```python
from build123d import *

# Parameters (mm, degrees)
SKETCH_R         = 2.5
PAD_DEPTH        = 80
SKETCH001_W      = 15
SKETCH001_H      = 10
POCKET_DEPTH     = 16
HOLE_D           = 4.5
HOLE_CSINK_D     = 10
HOLE_CSINK_ANGLE = 90
FILLET_R         = 4
FILLET001_R      = 2
CHAMFER_SIZE2    = 6
CHAMFER_SIZE     = 3
CHAMFER001_SIZE2 = 6
CHAMFER001_SIZE  = 3
FILLET002_R      = 1
FILLET003_R      = 1
FILLET004_R      = 2


with BuildPart() as part:
    # Sketch → Pad (new body)
    with BuildSketch(Plane.XY):
        Polygon((0, 0), (0, 15), (8.325291, 15), (16, 8), (30, 8), (30, 0), align=None)
        with Locations((6, 9)):
            Circle(SKETCH_R, mode=Mode.SUBTRACT)
    extrude(amount=PAD_DEPTH)

    # Sketch001 (on Face1 of Pad) → Pocket (cut)
    with BuildSketch(Plane(origin=(0, 0, 0), x_dir=(0, -1, 0), z_dir=(-1, 0, 0))):
        with Locations((-7.5, 15)):
            Rectangle(SKETCH001_W, SKETCH001_H)
        with Locations((-7.5, 35)):
            Rectangle(SKETCH001_W, SKETCH001_H)
        with Locations((-7.5, 55)):
            Rectangle(SKETCH001_W, SKETCH001_H)
        with Locations((-7.5, 75)):
            Rectangle(SKETCH001_W, SKETCH001_H)
    extrude(amount=-POCKET_DEPTH, mode=Mode.SUBTRACT)

    # Hole (through all)
    with Locations(Plane(origin=(0, 8, 0), x_dir=(-1, 0, 0), z_dir=(0, 1, 0))):
        with Locations((-22.5, 70), (-22.5, 50), (-22.5, 30), (-22.5, 10)):
            CounterSinkHole(HOLE_D / 2, HOLE_CSINK_D / 2, counter_sink_angle=HOLE_CSINK_ANGLE)

    # Fillet
    fillet_edges = [part.edges().sort_by_distance(p)[0] for p in [
        (0, 15, 5),
        (0, 15, 25),
        (0, 15, 45),
        (0, 15, 65),
    ]]
    fillet(fillet_edges, radius=FILLET_R)

    # Fillet001
    fillet001_edges = [part.edges().sort_by_distance(p)[0] for p in [
        (8.325291, 15, 5),
        (8.325291, 15, 25),
        (8.325291, 15, 45),
        (8.325291, 15, 65),
    ]]
    fillet(fillet001_edges, radius=FILLET001_R)

    # Chamfer
    chamfer_edges = [part.edges().sort_by_distance(p)[0] for p in [
        (0, 0, 25),
        (0, 0, 45),
        (0, 0, 65),
    ]]
    chamfer_side = part.faces().sort_by_distance((17.359651, 0, 38.113633))[0]
    chamfer(chamfer_edges, length=CHAMFER_SIZE, length2=CHAMFER_SIZE2, reference=chamfer_side)

    # Chamfer001
    chamfer001_edges = [part.edges().sort_by_distance(p)[0] for p in [
        (0, 0, 5),
    ]]
    chamfer001_side = part.faces().sort_by_distance((18.248211, 0, 37.727814))[0]
    chamfer(chamfer001_edges, length=CHAMFER001_SIZE, length2=CHAMFER001_SIZE2, reference=chamfer001_side)

    # Fillet002
    fillet002_edges = [part.edges().sort_by_distance(p)[0] for p in [
        (16, 8, 5),
        (16, 8, 25),
        (16, 8, 45),
        (16, 8, 65),
    ]]
    fillet(fillet002_edges, radius=FILLET002_R)

    # Fillet003
    fillet003_edges = [part.edges().sort_by_distance(p)[0] for p in [
        (16, 4, 10),
        (16, 4, 30),
        (16, 4, 50),
        (16, 4, 70),
        (16, 4, 80),
        (16, 4, 20),
        (16, 4, 40),
        (16, 4, 60),
    ]]
    fillet(fillet003_edges, radius=FILLET003_R)

    # Fillet004
    fillet004_edges = [part.edges().sort_by_distance(p)[0] for p in [
        (30, 4, 0),
        (30, 4, 80),
    ]]
    fillet(fillet004_edges, radius=FILLET004_R)


solid = part.part
```
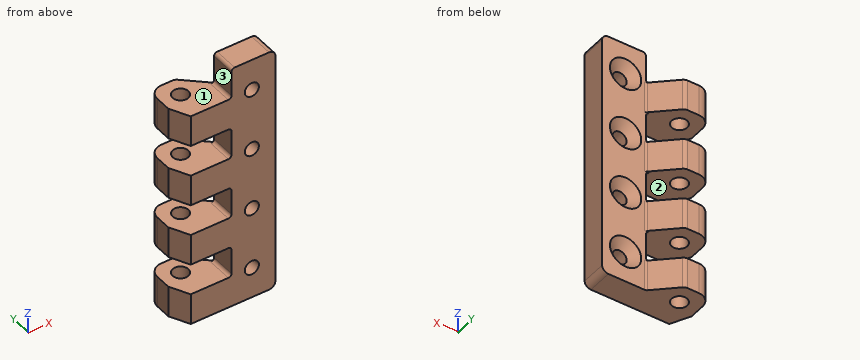
For this review, take the finished solid that the model builds, in its own axes (mm). Face numbers are marked on the shaded views. Round coordinates to 2 decimals unless told otherwise and drop trailing zeros. Write each loop counter-clockwise with the first axis right and the second up, starting at its lowest first coordinate (ties: lowest second). Pieces come first, ordered by that corner, then holes. Notation, with made-up numbers: (-31, 48) - (20, 48) arc R16 ccw to (20, 55) - close; hole circle Ø11 at (-34, 41.5). An arc over 180 degrees is marked (long way). Answer as a JSON object with one key per item and string values.
1. We need section A-A on x = 22.5. Give the boundary of the cut face in (y, z).
Response values:
{"outline": "(0, 0) - (8, 0) - (8, 5) - (5.25, 7.75) - (0, 7.75) - close; (0, 12.25) - (5.25, 12.25) - (8, 15) - (8, 25) - (5.25, 27.75) - (0, 27.75) - close; (0, 32.25) - (5.25, 32.25) - (8, 35) - (8, 45) - (5.25, 47.75) - (0, 47.75) - close; (0, 52.25) - (5.25, 52.25) - (8, 55) - (8, 65) - (5.25, 67.75) - (0, 67.75) - close; (0, 72.25) - (5.25, 72.25) - (8, 75) - (8, 80) - (0, 80) - close"}
2. We need section C-C on y = 3. Count the separate pieces of the cut face and the enclosed holes in it, then the cut area to 3 significant figures.
Response values:
{"separate pieces": "1", "enclosed holes": "4", "area": "1,640 mm2"}
3. To check wall thickness, follow line 1 along Z through (x, y) = (22.5, 4.25); line 2 along Z through (x, y) = (11.5, 7); line 3 along Y through (x, z) = (6, 4.75). State the ranges of each line that lie inside material, in increasing order.
Response values:
{"line 1": "z = 0 to 7.75, 12.25 to 27.75, 32.25 to 47.75, 52.25 to 67.75, 72.25 to 80", "line 2": "z = 0 to 10, 20 to 30, 40 to 50, 60 to 70", "line 3": "y = 0 to 6.5, 11.5 to 15"}
4. We need section B-B on z = 44. Give the boundary of the cut face in (x, y), then the cut area to 3 significant figures.
Response values:
{"outline": "(0, 6) - (3, 0) - (30, 0) - (30, 8) - (16.39, 8) arc R1 cw to (15.71, 8.26) - (8.9, 14.48) arc R2 ccw to (7.55, 15) - (4, 15) arc R4 ccw to (0, 11) - close; hole circle Ø5 at (6, 9)", "area": "293 mm2"}
5. Draft analysis for pull direction Z (two halves, no side actions). For the marked faces 1, 2 and 3, state which applies: +Z half, -Z half, draft (parallel to the pull), parting line (faces both ways), or undercut.
Response values:
{"face 1": "+Z half", "face 2": "undercut", "face 3": "draft"}
6. For pin 1 Ø4 at (y, z) = (4, 76.5) entering from -X; pin 2 Ø4.5 at (x, y) = (6, 11) entering from +Z; pin 3 Ø7 at (x, z) = (22.5, 50) entering from +Y, all flat-tipped, find the tip position at first contact; note any pin that passes through.
Response values:
{"pin 1": "stops at x = 16", "pin 2": "stops at z = 70", "pin 3": "stops at y = 6.5"}
